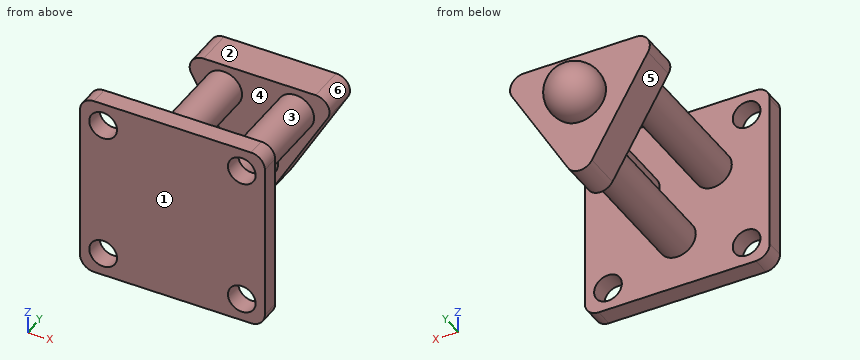
```python
from build123d import *
from build123d.topology import SkipClean

# Parameters (mm, degrees)
SKETCH_1_R      = 1.5
EXTRUDE_1_DEPTH = 2
SKETCH_2_R      = 2
EXTRUDE_2_DEPTH = 15
EXTRUDE_3_DEPTH = 4


with BuildPart() as part:
    # Sketch 1 → Extrude 1 (new body)
    with BuildSketch(Plane(origin=(0, 0, 0), x_dir=(1, 0, 0), z_dir=(0, 1, 0))):
        with BuildLine():
            Line((-8.5, -10), (8.5, -10))
            ThreePointArc((8.5, -10), (9.560660172, -9.560660172), (10, -8.5))
            Line((10, -8.5), (10, 8.5))
            ThreePointArc((10, 8.5), (9.560660172, 9.560660172), (8.5, 10))
            Line((8.5, 10), (-8.5, 10))
            ThreePointArc((-8.5, 10), (-9.560660172, 9.560660172), (-10, 8.5))
            Line((-10, 8.5), (-10, -8.5))
            ThreePointArc((-10, -8.5), (-9.560660172, -9.560660172), (-8.5, -10))
        make_face()
        with Locations(Location((7.5, 7.5, 0), (0, 0, 270))):
            Circle(SKETCH_1_R, mode=Mode.SUBTRACT)
        with Locations(Location((-7.5, 7.5, 0), (0, 0, 270))):
            Circle(SKETCH_1_R, mode=Mode.SUBTRACT)
        with Locations(Location((-7.5, -7.5, 0), (0, 0, 270))):
            Circle(SKETCH_1_R, mode=Mode.SUBTRACT)
        with Locations(Location((7.5, -7.5, 0), (0, 0, 270))):
            Circle(SKETCH_1_R, mode=Mode.SUBTRACT)
    extrude(amount=EXTRUDE_1_DEPTH)

    # Sketch 2 → Extrude 2 (add)
    with BuildSketch(Plane(origin=(0, 2, 0), x_dir=(1, 0, 0), z_dir=(0, 1, 0))):
        with Locations(Location((0, 4.5, 0), (0, 0, 90))):
            Circle(SKETCH_2_R)
        with Locations(Location((3.897114317, -2.25, 0), (0, 0, 90))):
            Circle(SKETCH_2_R)
        with Locations(Location((-3.897114317, -2.25, 0), (0, 0, 90))):
            Circle(SKETCH_2_R)
    extrude(amount=EXTRUDE_2_DEPTH)

    # Sketch 4 → Extrude 3 (add)
    with BuildSketch(Plane(origin=(0, 17, 0), x_dir=(1, 0, 0), z_dir=(0, 1, 0))):
        with BuildLine():
            Line((-1.299038106, 7.75), (-7.361215932, -2.75))
            ThreePointArc((-7.361215932, -2.75), (-7.361215932, -4.25), (-6.062177826, -5))
            Line((-6.062177826, -5), (6.062177826, -5))
            ThreePointArc((6.062177826, -5), (7.361215932, -4.25), (7.361215932, -2.75))
            Line((7.361215932, -2.75), (1.299038106, 7.75))
            ThreePointArc((1.299038106, 7.75), (0, 8.5), (-1.299038106, 7.75))
        make_face()
    extrude(amount=EXTRUDE_3_DEPTH)

    # Sketch 7 → Revolve 4 (revolve)
    with SkipClean():  # the faces are left unmerged after this step: merging them gives an invalid solid
        with BuildSketch(Plane.XY, mode=Mode.PRIVATE) as revolve_4_sk:
            with BuildLine():
                ThreePointArc((0, 25), (-3, 22), (0, 19))
                Line((0, 19), (0, 25))
            make_face()
            with BuildLine():
                Line((0, 25), (0, 19))
                ThreePointArc((0, 19), (2.121320344, 19.878679656), (3, 22))
                ThreePointArc((3, 22), (2.121320344, 24.121320344), (0, 25))
            make_face()
        revolve(revolve_4_sk.sketch.rotate(Axis((0, 19, 0), (0, 1, 0)), 180), axis=Axis((0, 19, 0), (0, 1, 0)))
    add(part.part.scale(1), mode=Mode.REPLACE)  # the faces are merged on a copy


solid = part.part
```
Verification items for the finished model (mm, model axes). Face numbers are marked on the shaded views. A direction names the side the tool comes from. Round coordinates to 2 decimals unless told otherwise and drop trailing zeros. Order: outer loops, then holes, each group sorted by start corner. A loop starts at its lowest first (then second) coordinate and runs counter-clockwise, first axis right, second up. Notation, with made-up numbers: (32, -38) - (42, -38) arc R25 cw to (42, -21) - close; hole circle Ø1 at (55, -7.5). An arc over 180 degrees is marked (long way). Use CSV: the item, a comma, the result in double quotes. Start each with the question number.
1) Section check C-C, the plane x = -5. Record the cut outline in (y, z), plus the area to 3 significant figures.
2) Go/stop test with flat-tipped pins: P1, Ø8, axis at x = -4, y = 20, coming from the +Z side; P2, Ø1.5, axis at y = 7, z = -2.5, coming from the -X side; P3, Ø10, axis at y = 21.5, z = 6.5, coming from the -X side. Record where each tip stops, or that it passes through.
3) Access from +Z, -Z, +X, -X, +Y, -Y to the whole of each face (thin tool, end or side, straight path). Record for the marked faces 4, 5 and 6.
4) Section check B-B, the plane y = 14. Record the cut outline in (x, z), plus the area to 3 significant figures.
5) Mould release check, pull along Y, two halves, no side actions. Record for the marked faces 1, 2 and 3: +Y half, -Y half, draft (parallel to the pull), parting line (faces both ways), or undercut.
6) Section check A-A, the plane z = 7.5. Record the cut outline in (x, y), plus the area to 3 significant figures.
7) Thickness scan on L1, parallel to X at y = 1.05, z = 7.5; L2, parallel to Y at x = -3.5, z = -2; L3, parallel to Y at x = -5.75, z = 8.75. Record the ranges inside material, lowest first.
8) Section check D-D, the plane z = -4.5. Record the cut outline in (x, y).
Answers:
1,outline,"(0, -10) - (2, -10) - (2, 0.58) - (17, 0.58) - (17, -1.34) - (21, -1.34) - (21, 5) - (17, 5) - (17, 3.92) - (2, 3.92) - (2, 10) - (0, 10) - close"
1,area,"115 mm²"
2,P1,"stops at z = 5"
2,P2,"stops at x = -1.56"
2,P3,"stops at x = -7.56"
3,face 4,"none"
3,face 5,"-Z, -X, +Y"
3,face 6,"+X, +Y"
4,outline,"circle Ø4 at (-3.9, 2.25); circle Ø4 at (0, -4.5); circle Ø4 at (3.9, 2.25)"
4,area,"37.7 mm²"
5,face 1,"-Y half"
5,face 2,"draft"
5,face 3,"undercut"
6,outline,"(-10, 0) - (-9, 0) - (-9, 2) - (-10, 2) - close; (-6, 0) - (6, 0) - (6, 2) - (-6, 2) - close; (9, 0) - (10, 0) - (10, 2) - (9, 2) - close"
6,area,"28.0 mm²"
7,L1,"x = -10 to -9, -6 to 6, 9 to 10"
7,L2,"y = 0 to 2, 17 to 21"
7,L3,"y = 0 to 2"
8,outline,"(-10, 0) - (10, 0) - (10, 2) - (2, 2) - (2, 17) - (3.18, 17) - (3.18, 21) - (-3.18, 21) - (-3.18, 17) - (-2, 17) - (-2, 2) - (-10, 2) - close"
